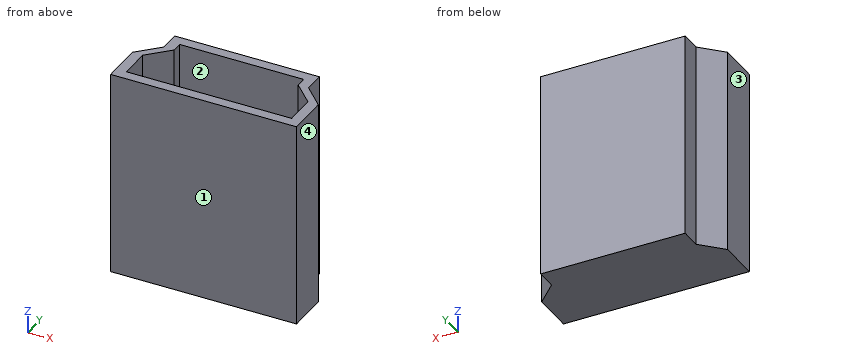
```python
from build123d import *

# Parameters (mm, degrees)
F0_W     = 7.14375
F0_H     = 7.9375
F1_DEPTH = 3.175
F3_DEPTH = 7.9385
F5_DEPTH = 7.62


with BuildPart() as f1:
    # F0 (on Front) → F1 (new body)
    with BuildSketch(Plane.XZ):
        with Locations((-18.391654, -5.990053)):
            Rectangle(F0_W, F0_H)
    extrude(amount=F1_DEPTH)

    # F2 (on face) → F3 (cut, through all)
    with BuildSketch(Plane(origin=(0, 0, -9.958803), x_dir=(1, 0, 0), z_dir=(0, 0, -1))):
        Polygon((-21.963529, 0), (-21.169779, 0), (-21.169779, 0.79375), (-21.963529, 1.5875), align=None)
        Polygon((-14.819779, 0), (-14.819779, 1.5875), (-15.613529, 0.79375), (-15.613529, 0), align=None)
    extrude(amount=-F3_DEPTH, mode=Mode.SUBTRACT)

    # F4 (on face) → F5 (cut)
    with BuildSketch(Plane.XY.offset(-2.021303)):
        Polygon((-21.566654, -2.778125), (-15.216654, -2.778125), (-15.216654, -1.5875), (-16.010404, -0.79375), (-16.010404, -0.396875), (-20.772904, -0.396875), (-20.772904, -0.79375), (-21.566654, -1.5875), align=None)
    extrude(amount=-F5_DEPTH, mode=Mode.SUBTRACT)


solid = f1.part
```
Model file for the job. Use its own axes, mm. Face numbers are marked on the shaded views. Give positions to 0.01 mm unless a question says otherwise; leave off trailing zeros. Loops run counter-clockwise (first coordinate to the right, second up) from the corner with the lowest first, then second, coordinate; pieces in that order, holes last. Notation, with made-up numbers: (35, -17.75) - (53, -17.75) arc R10 ccw to (53, -7.75) - close; hole circle Ø11 at (61, 0.25). An arc over 180 degrees is marked (long way). One line per item, written item: value. Start each with the question number.
1. Probe L1, parallel to Y at x = -18, z = -9 (3 decimals); L2, parallel to X at y = -1.75, z = -5.75; L3, parallel to Z at x = -19, y = -2.6. List the from-to ranges inside material, lowest first. Write a range as from..to.
2. Pull direction X, two halves, no side cores. Call the marked faces 1, 2, 3 and 4: pulls with the +X half, pulls with the -X half, needs draft (parallel to the pull), parting line crosses it, or undercut.
3. Slice it at B-B (y = -2.5). List the corners of the cut face in (x, z).
4. Slice it at C-C (x = -16.5). List the corners of the cut face in (y, z) (3 decimals).
5. Pin check, flat tip, straight feed: pin 1 (0.7 mm diameter, centred on x = -19.5, y = -2, fed in from +Z). Stop position of the tip, or through.
Solution:
1. L1: y = -3.175..-2.778, -0.397..0
1. L2: x = -21.96..-21.57, -15.22..-14.82
1. L3: z = -9.96..-9.64
2. face 1: needs draft
2. face 2: undercut
2. face 3: pulls with the -X half
2. face 4: pulls with the +X half
3. outline: (-21.96, -9.96) - (-14.82, -9.96) - (-14.82, -2.02) - (-15.22, -2.02) - (-15.22, -9.64) - (-21.57, -9.64) - (-21.57, -2.02) - (-21.96, -2.02) - close
4. outline: (-3.175, -9.959) - (0, -9.959) - (0, -2.021) - (-0.397, -2.021) - (-0.397, -9.641) - (-2.778, -9.641) - (-2.778, -2.021) - (-3.175, -2.021) - close
5. pin 1: stops at z = -9.64
